For this review, take the finished solid that the model builds, in its own axes (mm). A direction names the side the tool comes from. Coordinates: 2 decimals unless noted, no trailing zeros. Order: outer loops, then holes, each group sorted by start corner. A loop starts at its lowest first (then second) coordinate and runs counter-clockwise, first axis right, second up. Notation, with made-up numbers: (-4.75, 55) -> (11.25, 55) arc R18 cw to (11.25, 64) -> close; hole circle Ø11 at (73.25, 78). An arc over 180 degrees is marked (long way). Answer as a JSON object with one key per item and string values. Group by question number.
1) Add section B-B, the plane x = 59.5. Write out the cut boundary in (y, z).
2) Wall thickness on L1, parallel to Z at x = -49.5, y = 8; L2, parallel to X at y = 103.5, z = 23; L3, parallel to Y at x = 8.5, z = 15: over which ranges is each line inside the solid? List them lowest first.
3) Draft analysis for pull direction X (two halves, no side actions). For faces 3 (the flat face through (1, 65, -73.673)), 4 (the cylindrical face through (48.87, -6.34, 29.09)), 5 (the cylindrical face through (-0.21, -6.16, 72.26)), 6 (the flat face through (-36.046, -6.162, 51.051)), state which applies: +X half, -X half, draft (parallel to the pull), parting line (faces both ways), or undercut.
4) Add section D-D, the plane x = 43. Write out the cut boundary in (y, z), then the cut area to 3 significant figures.
5) Machinability: for faces 1 (the flat face through (-1, 140, -24)), 2 (the flat face through (1, 0, 38)), which of the approach directions +Z, -Z, +X, -X, +Y, -Y give a long, thin tool a straight path to every point of the face, cutting with its end or side? Answer none if there is none.
6) Add section A-A, the plane y = 59.5. Write out the cut boundary in (x, z).
7) For pin 1 (12.5 mm diameter, centred on x = -59, y = 46, fed in from +Z); pin 2 (1 mm diameter, centred on x = 40.5, y = 28.5, fed in from +Z), all flat-tipped, find the tip position at first contact; note any pin that passes through.
8) Add section C-C, the plane z = 39. Write out the cut boundary in (x, y), then the cut area to 3 significant figures.
from build123d import *

# Parameters (mm, degrees)
BOSS_EXTRUDE1_DEPTH = 140
BOSS_EXTRUDE2_DEPTH = 12.5
FILLET1_R           = 10


with BuildPart() as part:
    # Sketch1 → Boss-Extrude1 (new body)
    with BuildSketch(Plane(origin=(0, 0, 0), x_dir=(1, 0, 0), z_dir=(0, 1, 0))):
        Polygon((0, 0), (47.891204829, -27.65), (73.3, -27.65), (73.3, 73.672860643), (-73.3, 73.672860643), (-73.3, -27.65), (-47.891204829, -27.65), align=None)
    extrude(amount=BOSS_EXTRUDE1_DEPTH)

    # Sketch3 → Boss-Extrude2 (add)
    with BuildSketch(Plane.XZ):
        with BuildLine():
            Line((-47.891204829, 27.65), (-22.581478328, 77.65))
            ThreePointArc((-22.581478328, 77.65), (0, 72.260277252), (22.581478328, 77.65))
            Line((22.581478328, 77.65), (47.891204829, 27.65))
            Line((47.891204829, 27.65), (73.3, 27.65))
            Line((73.3, 27.65), (73.3, -73.672860643))
            Line((73.3, -73.672860643), (-73.3, -73.672860643))
            Line((-73.3, -73.672860643), (-73.3, 27.65))
            Line((-73.3, 27.65), (-47.891204829, 27.65))
        make_face()
    extrude(amount=BOSS_EXTRUDE2_DEPTH)

    # Fillet1
    fillet1_edges = [part.edges().sort_by_distance(p)[0] for p in [
        (-47.891204829, -6.25, 27.65),
        (47.891204829, -6.25, 27.65),
        (22.581478328, -6.25, 77.65),
        (-22.581478328, -6.25, 77.65),
    ]]
    fillet(fillet1_edges, radius=FILLET1_R)


solid = part.part
Output values:
{
 "1": {"outline": "(-12.5, -73.67) -> (140, -73.67) -> (140, 27.65) -> (-12.5, 27.65) -> close"},
 "2": {"L1": "z = -73.67 to 27.65", "L2": "x = -73.3 to -39.84, 39.84 to 73.3", "L3": "y = -12.5 to 0"},
 "3": {"face 3": "draft", "face 4": "+X half", "face 5": "undercut", "face 6": "-X half"},
 "4": {"outline": "(-12.5, -73.67) -> (140, -73.67) -> (140, 24.83) -> (0, 24.83) -> (0, 37.31) -> (-12.5, 37.31) -> close", "area": "15,200 mm²"},
 "5": {"face 1": "+Z, -Z, +X, -X, +Y", "face 2": "+Z, +Y"},
 "6": {"outline": "(-73.3, -73.67) -> (73.3, -73.67) -> (73.3, 27.65) -> (47.89, 27.65) -> (0, 0) -> (-47.89, 27.65) -> (-73.3, 27.65) -> close"},
 "7": {"pin 1": "stops at z = 27.65", "pin 2": "stops at z = 23.67"},
 "8": {"outline": "(-42.15, -12.5) -> (42.15, -12.5) -> (42.15, 0) -> (-42.15, 0) -> close", "area": "1,050 mm²"}
}
